Can you work these out from the model? Positions are in its coordinate system, mm. Give positions to 0.01 mm unless a question says otherwise; leave off trailing zeros. Order: outer loops, then holes, each group sorted by start corner. A loop starts at its lowest first (then second) coordinate and runs counter-clockwise, first axis right, second up. Notation, with made-up numbers: (29.5, 41.5) - (52.5, 41.5) arc R18 ccw to (52.5, 50.5) - close; hole circle Ø2 at (-1, 26). An arc over 180 degrees is marked (long way). Return JSON: item names as keys, results as strings.
```python
from build123d import *

# Parameters (mm, degrees)
SKETCH3_R = 0.5969


with BuildPart() as part:
    # Sweep1: sweep along a path in Sketch4
    with BuildLine(Plane(origin=(0, 0, 0), x_dir=(0, 0, -1), z_dir=(1, 0, 0))) as sweep1_path:
        Line((-18.57375, 4.859208931), (-7.776103247, -1.374815329))
        ThreePointArc((-7.776103247, -1.374815329), (-6.771462378, -1.573429786), (-5.854582736, -1.117268957))
        ThreePointArc((-5.854582736, -1.117268957), (-3.175, 0), (-0.495417264, -1.117268957))
        ThreePointArc((-0.495417264, -1.117268957), (0.28573535, -1.549197303), (1.176473152, -1.491338251))
        Line((1.176473152, -1.491338251), (14.975871107, 3.543419685))
        ThreePointArc((14.975871107, 3.543419685), (19.983040744, 0.656431604), (16.2687, -3.7719))
        Line((16.2687, -3.7719), (-20.6375, -3.7719))
    # Sketch3 → Sweep1 (sweep)
    with BuildSketch(Plane.XY.offset(20.6375)):
        with Locations((0, -3.7719)):
            Circle(SKETCH3_R)
    sweep(path=sweep1_path.line)


solid = part.part
```
1. Suppose I cut it at A-A (x = 0.4). List the corners of the cut face in (y, z) for me (1 decimal).
Checks:
{"outline": "(-4.2, -16.3) arc R4.2 ccw (long way) to (4, -14.8) - (-1.1, -1) arc R1.1 cw to (-0.8, 0.2) arc R4.2 ccw to (-0.8, 6.2) arc R1.1 cw to (-1, 7.6) - (5.2, 18.4) - (4.5, 18.8) - (-1.8, 8) arc R2 ccw to (-1.4, 5.5) arc R3.3 cw to (-1.4, 0.8) arc R2 ccw to (-1.9, -1.3) - (3.1, -15.1) arc R3.3 cw (long way) to (-3.3, -16.3) - (-3.3, 20.6) - (-4.2, 20.6) - close"}
2. If I drill on L1, parallel to Y at x = -0.15, z = 5; L2, parallel to Y at x = 0, z = 12 (3 decimals); L3, parallel to Z at x = 0.3, y = -2.5, over which ranges is the centre line in solid material (lowest first)? Write a range as [from, to].
Checks:
{"L1": "[-4.35, -3.19], [-1.15, 0.18]", "L2": "[-4.369, -3.175], [0.375, 1.753]", "L3": "[-19.75, -18.35]"}
3. For pin 1 Ø5 at (y, z) = (-2, -6.5) entering from -X, with a flat end and sliding along its axis, tell me the tip position at first contact or that it passes through.
Checks:
{"pin 1": "x = -0.6"}
4. Thinking about a two-plate mould opening in Z: for faces 1 (the face through (0, -4, 20.638)), 2 (the face through (-0.08, -3.18, 2.44)), 3 (the face through (-0.078, 0.505, -8.376)), which applies, +Z half, -Z half, draft (parallel to the pull), parting line (faces both ways), or undercut?
Checks:
{"face 1": "+Z half", "face 2": "draft", "face 3": "undercut"}
